Autodesk Inventor part; units mm, degrees
ref_plane "YZ Plane" through (0, 0, 0) normal (1, 0, 0) x (0, 1, 0)
ref_plane "XZ Plane" through (0, 0, 0) normal (0, 1, 0) x (-1, 0, 0)
ref_plane "XY Plane" through (0, 0, 0) normal (0, 0, 1) x (1, 0, 0)
sketch "Schizzo1" plane through (0, 0, 0) normal (0, 0, 1) x (1, 0, 0)
  circle A0 centre (0, 0) radius 5.25
  arc A1 (9, 0) -> (-9, 0) centre (0, 0) ccw
  line L0 (-9, 0) -> (-9, -10)
  line L1 (-9, -10) -> (9, -10)
  line L2 (9, -10) -> (9, 0)
  dimension "d0" = 10.5
  dimension "d1" = 18
  dimension "d2" = 10
extrude "Piano1" add sketch "Schizzo1" along normal blind 3
sketch "Schizzo2" plane through (-9, -13, -3) normal (0, -1, 0) x (1, 0, 0)
  line L0 (18, 0) -> (0, 0)
  line L1 (0, 0) -> (0, -14)
  line L2 (0, -14) -> (18, -14)
  line L3 (18, -14) -> (18, 0)
edge flange "Flangia1" height 20 angle 90 thickness 3 bend radius 3 thickness toward (0, -1, 0) relief tear relief width 3 relief depth 1.5 edges at (0, -10, 0) wall of the first edge with corners at (9, -13, -3) (-9, -13, -3) (-9, -13, -17) (9, -13, -17)
bend "Piega (Bend)1"
corner "Angolo1"
fillet "Arrotondamento angolo1" radius 2 2 edges at (9, -14.5, -17) (-9, -14.5, -17)
equation "\"d3\" = Spessore"
equation "\"d4\" = LarghezzaScaricoPiega"
equation "\"d5\" = ProfonditàScaricoPiega"
equation "\"d6\" = ResiduoMinimo"
equation "\"d7\" = RaggioTransizione"
equation "\"d10\" = RaggioPiega"
equation "\"d11\" = DimensioniScaricoAngolo"
equation "\"d12\" = DimensioneGioco"
equation "\"d13\" = Dimensione_raggio_Jacobi"
equation "\"RaggioPiega\" = Spessore"
equation "\"LarghezzaScaricoPiega\" = Spessore"
equation "\"ProfonditàScaricoPiega\" = 0.5 * Spessore"
equation "\"DimensioniScaricoAngolo\" = 4 * Spessore"
equation "\"ResiduoMinimo\" = 2 * Spessore"
equation "\"RaggioTransizione\" = RaggioPiega"
equation "\"Dimensione_raggio_Jacobi\" = RaggioPiega"
equation "\"DimensioneGioco\" = Spessore"
properties part number "Supporto perno tendi motore" material "Acciaio inossidabile"
Work out the finished part from the listing and answer in its coordinate system (mm). A direction names the side the tool comes from. Round coordinates to 2 decimals unless told otherwise and drop trailing zeros. Write each loop counter-clockwise with the first axis right and the second up, starting at its lowest first coordinate (ties: lowest second). Pieces come first, ordered by that corner, then holes. Notation, with made-up numbers: (-32.5, 36.5) -> (-7.5, 36.5) arc R28 ccw to (-7.5, 63.5) -> close; hole circle Ø7 at (70.25, 8.25). An arc over 180 degrees is marked (long way). Write each question's results on one line, items separated by ' | '.
1) The part is cut by section B-B (z = -8). Write down the section's boundary in (x, y), and give its area (3 significant figures).
Findings:
outline: (-9, -16) -> (9, -16) -> (9, -13) -> (-9, -13) -> close | area: 54.0 mm²
2) The part is cut by section A-A (x = 0). Write down the section's boundary in (y, z), and give its area (3 significant figures).
Findings:
outline: (-16, -17) -> (-13, -17) -> (-13, -3) arc R3 cw to (-10, 0) -> (-5.25, 0) -> (-5.25, 3) -> (-10, 3) arc R6 ccw to (-16, -3) -> close; (5.25, 0) -> (9, 0) -> (9, 3) -> (5.25, 3) -> close | area: 88.7 mm²
3) For a pull along X with two mould halves and no side action, classify faces 1 (the cylindrical face through (-0.13, -12.14, -0.9)), 2 (the flat face through (-9, -13.3, -3.4)), 3 (the cylindrical face through (5, -1.6, 1.5)) as +X half, -X half, draft (parallel to the pull), parting line (faces both ways), or undercut.
Findings:
face 1: draft | face 2: -X half | face 3: undercut
4) The part is cut by section D-D (y = 6.5). Write down the section's boundary in (x, z).
Findings:
outline: (-6.22, 0) -> (6.22, 0) -> (6.22, 3) -> (-6.22, 3) -> close
5) Which of the six approach directions +Z, -Z, +X, -X, +Y, -Y give full straight-line access (tool end or side, diameter ignored) to faces 4 (the cylindrical face through (-8.43, -14.52, -16.4)), 5 (the flat face through (0, -13, -10))?
Findings:
face 4: -Z, -X, +Y, -Y | face 5: -Z, +X, -X, +Y
6) Consider line 1 along Y through (x, z) = (5.25, -6.75); line 2 along Z through (x, y) = (-6.5, -1); line 3 along Y through (x, z) = (0, 2.05). Determine where each line is inside the solid, lowest interval first. Write a range as [from, to].
Findings:
line 1: y = [-16, -13] | line 2: z = [0, 3] | line 3: y = [-13.24, -5.25], [5.25, 9]
7) Flat-ended cylindrical pins translate along their axes: pin 1 (12 mm diameter, centred on y = 5, z = -3.5, fed in from -X); pin 2 (6 mm diameter, centred on y = 4, z = -1, fed in from +X); pin 3 (7 mm diameter, centred on x = 2, z = -6.5, fed in from +Y); pin 4 (1 mm diameter, centred on x = -3, y = -10.5, fed in from +Z). Find the tip coordinate at first contact, or state that the pin passes through.
Findings:
pin 1: stops at x = -9 | pin 2: stops at x = 8.92 | pin 3: stops at y = -13 | pin 4: stops at z = 3
8) The part is cut by section C-C (x = 6). Write down the section's boundary in (y, z), and give its area (3 significant figures).
Findings:
outline: (-16, -17) -> (-13, -17) -> (-13, -3) arc R3 cw to (-10, 0) -> (6.71, 0) -> (6.71, 3) -> (-10, 3) arc R6 ccw to (-16, -3) -> close | area: 113 mm²
